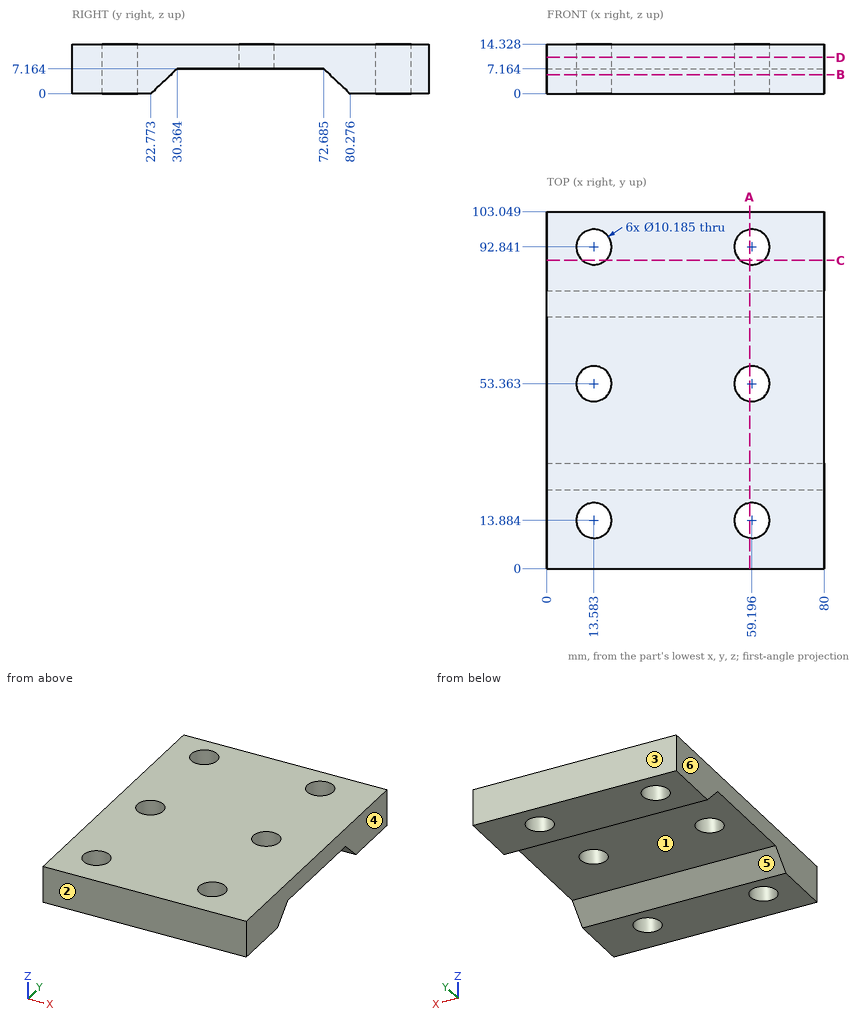
Could you check a few things on this drawing? It's one solid part, dimensions in mm from its lowest x, y, z. A direction names the side the tool comes from. Give positions to 0.01 mm unless a question says otherwise; leave off trailing zeros. Write each loop counter-clockwise with the first axis right and the second up, starting at its lowest first coordinate (ties: lowest second). Pieces come first, ordered by that corner, then holes. Notation, with made-up numbers: M 57,10.25 L 106,10.25 A32 cw 106,45.25 Z; hole C 71.5,24 d9. An arc over 180 degrees is marked long. Put each result on its own line as item: value. Start each with the question number.
Item 1: If we section it at C-C, the plane y = 89: Write out the boundary of the cut face in (x, z).
Item 2: On a 3-axis mill with a long thin cutter (end or side, diameter ignored), from which of +Z, -Z, +X, -X, +Y, -Y can I reach the whole of each face in a straight line? I mean the marked faces 5 and 6. Say none if no direction works.
Item 3: If we section it at B-B, the plane z = 5.5: Write out the boundary of the cut face in (x, y) (1 decimal).
Item 4: If we section it at A-A, the plane x = 58.5: Write out the boundary of the cut face in (y, z) (1 decimal).
Item 5: Thinking about a two-plate mould opening in Y: for the marked faces 1, 2, 3 and 4, which applies, +Y half, -Y half, draft (parallel to the pull), parting line (faces both ways), or undercut?
Item 6: I need wall thicknesses on L1, parallel to Y at x = 58.5, z = 12.25 (1 decimal); L2, parallel to X at y = 16.5, z = 5.5 (1 decimal); L3, parallel to Z at x = 46.5, y = 50. Which ranges of each line are inside material? Lowest first, please. Write a range as from..to.
Item 7: Will these pins go through, and if not, where does the flat tip stop? pin 1 (6 mm diameter, centred on x = 59.2, y = 53.36, fed in from -Z); pin 2 (5 mm diameter, centred on y = 23.5, z = 2, fed in from -X).
Item 8: If we section it at D-D, the plane z = 10.5: Write out the boundary of the cut face in (x, y) (1 decimal).
Values:
1. outline: M 0,0 L 10.24,0 L 10.24,14.33 L 0,14.33 Z; M 16.93,0 L 55.85,0 L 55.85,14.33 L 16.93,14.33 Z; M 62.54,0 L 80,0 L 80,14.33 L 62.54,14.33 Z
2. face 5: -Z, +X, -X
2. face 6: +Z, -Z, -X, +Y, -Y
3. outline: M 0,0 L 80,0 L 80,28.6 L 0,28.6 Z; M 0,74.4 L 80,74.4 L 80,103 L 0,103 Z; hole C 13.6,13.9 d10.2; hole C 13.6,92.8 d10.2; hole C 59.2,13.9 d10.2; hole C 59.2,92.8 d10.2
4. outline: M 0,0 L 8.8,0 L 8.8,14.3 L 0,14.3 Z; M 18.9,0 L 22.8,0 L 30.4,7.2 L 48.3,7.2 L 48.3,14.3 L 18.9,14.3 Z; M 58.4,7.2 L 72.7,7.2 L 80.3,0 L 87.8,0 L 87.8,14.3 L 58.4,14.3 Z; M 97.9,0 L 103,0 L 103,14.3 L 97.9,14.3 Z
5. face 1: undercut
5. face 2: -Y half
5. face 3: +Y half
5. face 4: draft
6. L1: 0..8.8, 18.9..48.3, 58.4..87.8, 97.9..103
6. L2: 0..9.2, 18..54.8, 63.6..80
6. L3: 7.16..14.33
7. pin 1: through
7. pin 2: x = 0
8. outline: M 0,0 L 80,0 L 80,103 L 0,103 Z; hole C 13.6,13.9 d10.2; hole C 13.6,53.4 d10.2; hole C 13.6,92.8 d10.2; hole C 59.2,13.9 d10.2; hole C 59.2,53.4 d10.2; hole C 59.2,92.8 d10.2
